from build123d import *

# Parameters (mm, degrees)
F0_W     = 1244.6
F0_H     = 698.5
F2_DEPTH = 2419.35
F3_W     = 838.2
F3_H     = 1524
F4_DEPTH = 698.5
F5_W     = 584.2
F5_H     = 1524
F6_DEPTH = 203.2
F7_W     = 838.2
F7_H     = 285.75
F8_DEPTH = 698.5


with BuildPart() as f2:
    # F0 (on Top) → F2 (new body)
    with BuildSketch(Plane.XY):
        Rectangle(F0_W, F0_H)
    extrude(amount=F2_DEPTH)

    # F3 (on face) → F4 (cut)
    with BuildSketch(Plane.XZ.offset(349.25)):
        with Locations((0, 1352.55)):
            Rectangle(F3_W, F3_H)
    extrude(amount=-F4_DEPTH, mode=Mode.SUBTRACT)

    # F5 (on face) → F6 (cut)
    with BuildSketch(Plane.YZ.offset(-419.1)):
        with Locations((57.15, 1352.55)):
            Rectangle(F5_W, F5_H)
    extrude(amount=-F6_DEPTH, mode=Mode.SUBTRACT)

    # F7 (on face) → F8 (cut)
    with BuildSketch(Plane.XZ.offset(349.25)):
        with Locations((0, 295.275)):
            Rectangle(F7_W, F7_H)
    extrude(amount=-F8_DEPTH, mode=Mode.SUBTRACT)


solid = f2.part
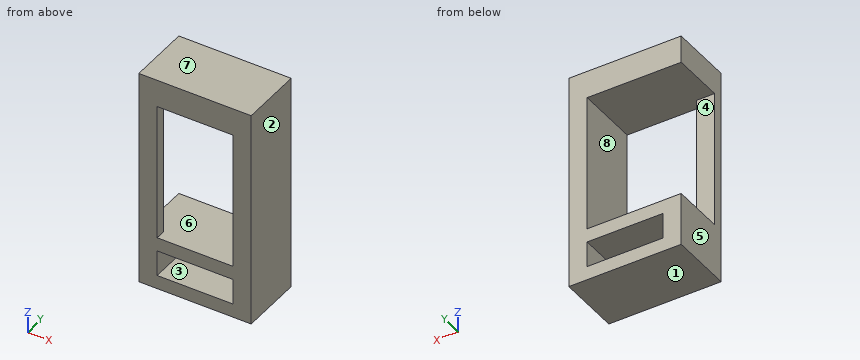
The model under review builds one solid part; all positions refer to its coordinate system, in mm. Face numbers are marked on the shaded views. A direction names the side the tool comes from. Round coordinates to 2 decimals unless told otherwise and drop trailing zeros. Loops run counter-clockwise (first coordinate to the right, second up) from the corner with the lowest first, then second, coordinate; pieces in that order, holes last. Notation, with made-up numbers: (1.25, -6) - (57.25, -6) arc R25 cw to (57.25, 20) - close; hole circle Ø6 at (-22.5, 55). An arc over 180 degrees is marked (long way). Use CSV: the item, a comma, the result in double quotes.
(1) Take a section at A-A, the plane y = -285. Give the boundary of the cut face in (x, z), plus the area to 3 significant figures.
Working result:
outline,"(-622.3, 0) - (622.3, 0) - (622.3, 2419.35) - (-622.3, 2419.35) - close; hole (-419.1, 152.4) - (419.1, 152.4) - (419.1, 438.15) - (-419.1, 438.15) - close; hole (-419.1, 590.55) - (419.1, 590.55) - (419.1, 2114.55) - (-419.1, 2114.55) - close"
area,"1,490,000 mm^2"
(2) Machinability: for the marked faces 4, 5, 6, 7 and 8, which of the approach directions +Z, -Z, +X, -X, +Y, -Y give a long, thin tool a straight path to every point of the face, cutting with its end or side? Answer none if there is none.
Working result:
face 4,"-X, +Y"
face 5,"+Z, -Z, -X, +Y, -Y"
face 6,"+Y"
face 7,"+Z, +X, -X, +Y, -Y"
face 8,"+Y, -Y"
(3) Take a section at B-B, the plane x = 308. Give the boundary of the cut face in (y, z).
Working result:
outline,"(-349.25, 0) - (349.25, 0) - (349.25, 152.4) - (-349.25, 152.4) - close; (-349.25, 438.15) - (349.25, 438.15) - (349.25, 590.55) - (-349.25, 590.55) - close; (-349.25, 2114.55) - (349.25, 2114.55) - (349.25, 2419.35) - (-349.25, 2419.35) - close"
(4) Take a section at D-D, the plane y = 292. Give the boundary of the cut face in (x, z), plus the area to 3 significant figures.
Working result:
outline,"(-622.3, 0) - (622.3, 0) - (622.3, 2419.35) - (-622.3, 2419.35) - (-622.3, 2114.55) - (419.1, 2114.55) - (419.1, 590.55) - (-622.3, 590.55) - close; hole (-419.1, 152.4) - (419.1, 152.4) - (419.1, 438.15) - (-419.1, 438.15) - close"
area,"1,180,000 mm^2"
(5) The part is to be moulded in two halves that separate along Z. For the marked faces 1, 2 and 3, say which applies: pulls with the +Z half, pulls with the -Z half, needs draft (parallel to the pull), parting line crosses it, or undercut.
Working result:
face 1,"pulls with the -Z half"
face 2,"needs draft"
face 3,"undercut"
(6) Clearance check with a flat-ended pin moving along its axis: P1, Ø1, axis at x = 12.5, y = -108.5, coming from the -Z side. State where the tip first meets the part, or that it passes through.
Working result:
P1,"stops at z = 0"
(7) For line 1 (Z direction, x = 372, y = 55); line 2 (X direction, y = -279, z = 1771); line 3 (X direction, y = -10.5, z = 1194), list the stretches that pass through material, from the lowest coordinate up.
Working result:
line 1,"z = 0 to 152.4, 438.15 to 590.55, 2114.55 to 2419.35"
line 2,"x = -622.3 to -419.1, 419.1 to 622.3"
line 3,"x = 419.1 to 622.3"
(8) Take a section at C-C, the plane z = 868. Give the boundary of the cut face in (x, y), plus the area to 3 significant figures.
Working result:
outline,"(-622.3, -349.25) - (-419.1, -349.25) - (-419.1, -234.95) - (-622.3, -234.95) - close; (419.1, -349.25) - (622.3, -349.25) - (622.3, 349.25) - (419.1, 349.25) - close"
area,"165,000 mm^2"
